Could you check a few things on this model? Use its own coordinates, in mm. A direction names the side the tool comes from. Give positions to 0.01 mm unless a question says otherwise; leave off trailing zeros. Order: outer loops, then holes, each group sorted by start corner. A loop starts at its lowest first (then second) coordinate and runs counter-clockwise, first axis right, second up.
from build123d import *

# Parameters (mm, degrees)
SKETCH4_R           = 7.9375
BOSS_EXTRUDE2_DEPTH = 12.7
SKETCH7_R           = 6.35
CUT_EXTRUDE2_DEPTH  = 12.7
SKETCH8_R           = 7.9375
BOSS_EXTRUDE4_DEPTH = 25.4
SKETCH10_R          = 6.35
CUT_EXTRUDE4_DEPTH  = 12.7
SKETCH9_R           = 6.35
CUT_EXTRUDE5_DEPTH  = 51.8


with BuildPart() as part:
    # Sketch4 → Boss-Extrude2 (new body)
    with BuildSketch(Plane.XY):
        Circle(SKETCH4_R)
    extrude(amount=BOSS_EXTRUDE2_DEPTH)

    # Sketch7 → Cut-Extrude2 (cut)
    with BuildSketch(Plane.XY.offset(12.7)):
        Circle(SKETCH7_R)
    extrude(amount=-CUT_EXTRUDE2_DEPTH, mode=Mode.SUBTRACT)

    # Sketch8 → Boss-Extrude4 (add, symmetric)
    with BuildSketch(Plane(origin=(0, 0, 0), x_dir=(0, 0, -1), z_dir=(1, 0, 0))):
        Circle(SKETCH8_R)
    extrude(amount=BOSS_EXTRUDE4_DEPTH, both=True)

    # Sketch10 → Cut-Extrude4 (cut)
    with BuildSketch(Plane.XY.offset(12.7)):
        Circle(SKETCH10_R)
    extrude(amount=-CUT_EXTRUDE4_DEPTH, mode=Mode.SUBTRACT)

    # Sketch9 → Cut-Extrude5 (cut, through all)
    with BuildSketch(Plane(origin=(25.4, 0, 0), x_dir=(0, 0, -1), z_dir=(1, 0, 0))):
        Circle(SKETCH9_R)
    extrude(amount=-CUT_EXTRUDE5_DEPTH, mode=Mode.SUBTRACT)


solid = part.part
Item 1: Imagine slicing it at A-A on y = 0. List the corners of the cut face in (x, z) for me.
Findings:
outline: (-25.4, -7.94) - (25.4, -7.94) - (25.4, -6.35) - (-25.4, -6.35) - close; (-25.4, 6.35) - (-6.35, 6.35) - (-6.35, 12.7) - (-7.94, 12.7) - (-7.94, 7.94) - (-25.4, 7.94) - close; (6.35, 6.35) - (25.4, 6.35) - (25.4, 7.94) - (7.94, 7.94) - (7.94, 12.7) - (6.35, 12.7) - close
Item 2: Please list where this line runs through material, in increasing order: line 1 along X through (y, z) = (0, 8.75).
Findings:
line 1: x = -7.94 to -6.35, 6.35 to 7.94
Item 3: For pin 1 (3 mm diameter, centred on x = 11.5, y = -2.5, fed in from +Z); pin 2 (1 mm diameter, centred on y = -3.5, z = 8.5, fed in from -X); pin 3 (4 mm diameter, centred on x = 4, y = -6.5, fed in from -Z), each with a flat end and sliding along its axis, tell me the tip position at first contact or that it passes through.
Findings:
pin 1: stops at z = 7.87
pin 2: stops at x = -7.35
pin 3: stops at z = -6.54
Item 4: We'd pull the mould along Y, two halves only. Please class faces 1 (the flat face through (0, 7, 12.7)), 2 (the cylindrical face through (0.356, 1.907, -6.057)), 3 (the cylindrical face through (0.356, 2.384, -7.571)): +Y half, -Y half, draft (parallel to the pull), parting line (faces both ways), or undercut.
Findings:
face 1: draft
face 2: undercut
face 3: parting line
Item 5: Imagine slicing it at D-D on y = 4. List the corners of the cut face in (x, z) for me, then the cut area to 3 significant figures.
Findings:
outline: (-25.4, -6.86) - (25.4, -6.86) - (25.4, -4.93) - (-25.4, -4.93) - close; (-25.4, 4.93) - (-4.93, 4.93) - (-4.93, 12.7) - (-6.86, 12.7) - (-6.86, 6.86) - (-25.4, 6.86) - close; (4.93, 4.93) - (25.4, 4.93) - (25.4, 6.86) - (6.86, 6.86) - (6.86, 12.7) - (4.93, 12.7) - close
area: 199 mm2
Item 6: For faces 4 (the flat face through (25.4, 7, 0)), 5 (the cylindrical face through (7.571, 2.384, 9.083)), which set-ups out of +Z, -Z, +X, -X, +Y, -Y let a thin tool reach every point of the face, with its end or its side?
Findings:
face 4: +Z, -Z, +X, +Y, -Y
face 5: +Z
